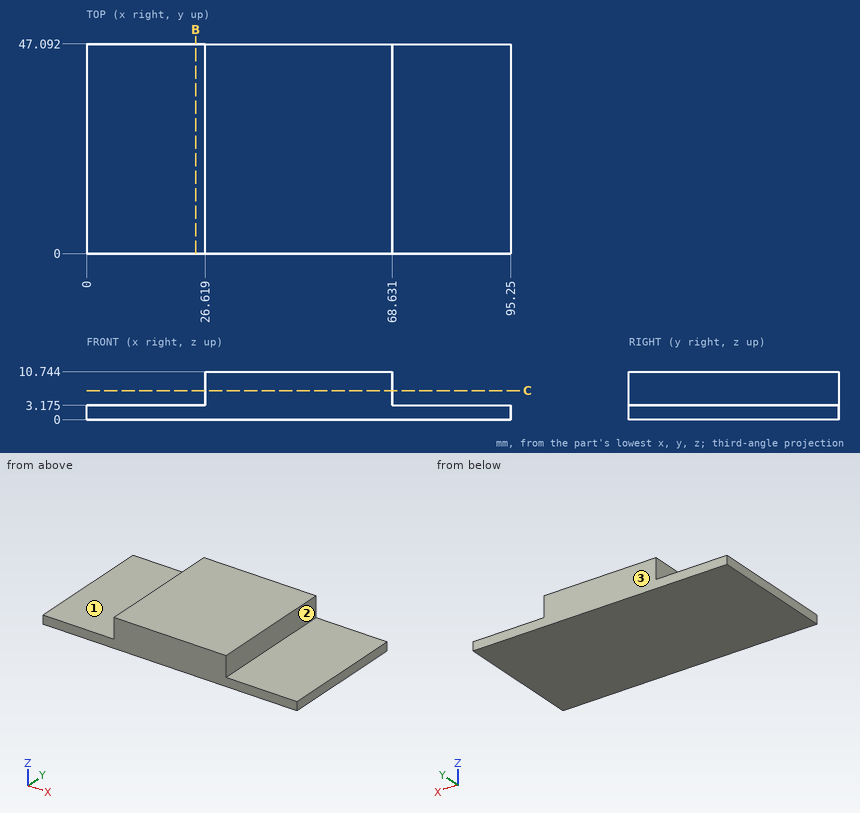
Answer from the drawing. Dimensions are ordinates in mm from the lowest x, y and z of the part. A direction names the side the tool comes from. Round coordinates to 2 decimals unless told otherwise and drop trailing zeros. Write each loop counter-clockwise with the first axis right and the second up, starting at its lowest first coordinate (ties: lowest second). Pieces come first, ordered by that corner, then holes. Notation, with made-up numbers: (66.25, 37.5) - (110.25, 37.5) arc R15 ccw to (110.25, 41.5) - close; hole circle Ø11 at (32.5, -13). An arc over 180 degrees is marked (long way). One line per item, written item: value.
Q1. Find section B-B (x = 24.5). Determine the outline of the cut face in (y, z) (1 decimal).
The answers:
outline: (0, 0) - (47.1, 0) - (47.1, 3.2) - (0, 3.2) - close
Q2. Straight lines are drawn through the part: line 1 (X direction, y = 7, z = 9.25); line 2 (Z direction, x = 25.5, y = 10) (1 decimal). For each, find the intervals that lie inside material, in ascending order. Write a range as from..to.
The answers:
line 1: x = 26.62..68.63
line 2: z = 0..3.2
Q3. Find section C-C (z = 6.5). Determine the outline of the cut face in (x, y), and give its area (3 significant figures).
The answers:
outline: (26.62, 0) - (68.63, 0) - (68.63, 47.09) - (26.62, 47.09) - close
area: 1,980 mm2
Q4. Each of these flat-tipped pins is pushed along its axis until it touches: P1, Ø13.5, axis at x = 80, y = 21, coming from the +Z side (3 decimals); P2, Ø4, axis at y = 12.5, z = 8.5, coming from the -X side. Where does it stop, or does it pass through?
The answers:
P1: stops at z = 3.175
P2: stops at x = 26.62
Q5. Which of the six approach directions +Z, -Z, +X, -X, +Y, -Y give full straight-line access (tool end or side, diameter ignored) to the marked faces 1, 2 and 3?
The answers:
face 1: +Z, -X, +Y, -Y
face 2: +Z, +X, +Y, -Y
face 3: +Z, -Z, +X, -X, +Y
